from build123d import *

# Parameters (mm, degrees)
BASE_EXTRUDE_DEPTH = 7.5


with BuildPart() as part:
    # Sketch1 → Base-Extrude (new body, symmetric)
    with BuildSketch(Plane.XY):
        with BuildLine():
            Line((0, 1.67), (0, 2))
            ThreePointArc((0, 2), (-1.414213562, -1.414213562), (2, 0))
            ThreePointArc((2, 0), (1.345868325, 1.249213562), (0, 1.67))
        make_face()
        with BuildLine():
            Line((-1.67, 0), (-1.34, 0))
            ThreePointArc((-1.34, 0), (-0.947523087, 0.947523087), (0, 1.34))
            ThreePointArc((0, 1.34), (1.112523087, 1.015868325), (1.67, 0))
            ThreePointArc((1.67, 0), (0, -1.67), (-1.67, 0))
        make_face(mode=Mode.SUBTRACT)
    extrude(amount=BASE_EXTRUDE_DEPTH, both=True)


solid = part.part
Work out the finished part from the listing and answer in its coordinate system (mm). Round coordinates to 2 decimals unless told otherwise and drop trailing zeros. Loops run counter-clockwise (first coordinate to the right, second up) from the corner with the lowest first, then second, coordinate; pieces in that order, holes last. Notation, with made-up numbers: (24.25, 39.5) - (48.25, 39.5) arc R6 ccw to (48.25, 43.5) - close; hole circle Ø10 at (-34, -13). An arc over 180 degrees is marked (long way). Use one line per item in the form item = value. Start each with the question number.
(1) Find section C-C on z = 5. Determine the outline of the cut face in (x, y) (3 decimals).
(2) Find section A-A on y = 0.95. Determine the outline of the cut face in (x, z).
(3) Find section B-B on x = 1.3. Determine the outline of the cut face in (y, z).
(4) Determine the mould class of faces 1 (the face through (0.04, -1.67, 0.11)), 2 (the face through (-1.46, -1.367, 0.105)) for opening direction X: +X half, -X half, draft (parallel to the pull), parting line (faces both ways), or undercut.
(5) Consider line 1 (Y direction, x = 0.65, z = 1.25); line 2 (Y direction, x = 0.9, z = -2); line 3 (X direction, y = 1.05, z = -4.25). Determine where each line is inside the solid, lowest interval first.
(6) Flat-ended cylindrical pins translate along their axes: P1, Ø1.5, axis at y = 1.5, z = -1, coming from the +X side; P2, Ø1, axis at x = -0.5, y = -1, coming from the -Z side. Find the tip coordinate at first contact, or state that the pin passes through.
Answer list:
q1.outline = (0, 1.67) - (0, 2) arc R2 ccw (long way) to (2, 0) arc R1.842 ccw to start; hole (-1.67, 0) arc R1.67 ccw to (1.67, 0) arc R1.514 ccw to (0, 1.34) arc R1.34 ccw to (-1.34, 0) - close
q2.outline = (-1.76, -7.5) - (-0.95, -7.5) - (-0.95, 7.5) - (-1.76, 7.5) - close; (1.19, -7.5) - (1.63, -7.5) - (1.63, 7.5) - (1.19, 7.5) - close
q3.outline = (-1.52, -7.5) - (-1.05, -7.5) - (-1.05, 7.5) - (-1.52, 7.5) - close; (0.84, -7.5) - (1.29, -7.5) - (1.29, 7.5) - (0.84, 7.5) - close
q4.face_1 = undercut
q4.face_2 = parting line
q5.line_1 = -1.89 to -1.54, 1.27 to 1.61
q5.line_2 = -1.79 to -1.41, 1.16 to 1.52
q5.line_3 = -1.7 to -0.83, 1.07 to 1.55
q6.P1 = 1.76
q6.P2 = through
